Part model, mm, in its own coordinate system. Face numbers are marked on the shaded views. A direction names the side the tool comes from. Coordinates: 2 decimals unless noted, no trailing zeros. Loops run counter-clockwise (first coordinate to the right, second up) from the corner with the lowest first, then second, coordinate; pieces in that order, holes last. Notation, with made-up numbers: (-6.5, -26) - (51.5, -26) arc R12 cw to (51.5, -9) - close; hole circle Ø9 at (38, -3). An arc over 180 degrees is marked (long way). Use a Markdown table: item, result. Add a question column.
1. Wall check: probe 1 along Y at (x, z) = (0, 7.75); probe 2 along X at (y, z) = (-2.5, 7); probe 3 along X at (y, z) = (-8.5, 6.5). Give the ranges that are in metal, low to high. Write a range as [from, to].
2. Band-saw the part on D-D, the plane z = 7.5. Give the cut face in (x, y), plus the area to 3 significant figures.
3. Band-saw the part on B-B, the plane y = 0. Give the cut face in (x, z).
4. Pull direction X, two halves, no side cores. Call the marked faces 1, 2 and 3: pulls with the +X half, pulls with the -X half, needs draft (parallel to the pull), parting line crosses it, or undercut.
5. Band-saw the part on C-C, the plane z = 2.75. Give the cut face in (x, y).
6. Drop flat-ended pins along their axis: pin 1 (5 mm diameter, centred on x = 21, z = 3.5, fed in from +Y); pin 2 (1 mm diameter, centred on y = -18, z = 3.5, fed in from +X); pin 3 (23.5 mm diameter, centred on x = 0, y = 0, fed in from +Z). Give the stop position or say it passes through.
7. 3-axis set-ups, long thin cutter, end or side, ignore diameter. For the marked faces 4 and 5: which of +Z, -Z, +X, -X, +Y, -Y reach the whole face in a straight line?
8. Band-saw the part on A-A, the plane x = 0. Give the cut face in (y, z), plus the area to 3 significant figures.
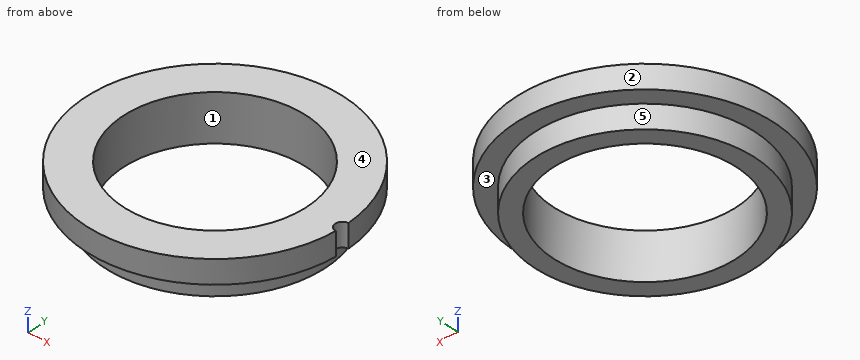
from build123d import *

# Parameters (mm, degrees)
SKETCH_R          = 27.5
SKETCH_R_2        = 19.5
PAD_DEPTH         = 10
SKETCH001_R       = 1.5
POCKET_DEPTH      = 10
SKETCH002_R       = 1.5
POCKET001_DEPTH   = 1.5
COPYSKETCH003_R   = 27.5
COPYSKETCH003_R_2 = 23.5
POCKET002_DEPTH   = 5


with BuildPart() as part:
    # Sketch → Pad (new body)
    with BuildSketch(Plane.XY):
        Circle(SKETCH_R)
        Circle(SKETCH_R_2, mode=Mode.SUBTRACT)
    extrude(amount=PAD_DEPTH)

    # Sketch001 → Pocket (cut)
    with BuildSketch(Plane(origin=(27.5, 0, 0), x_dir=(1, 0, 0), z_dir=(0, 0, 1))):
        Circle(SKETCH001_R)
    extrude(amount=POCKET_DEPTH, mode=Mode.SUBTRACT)

    # Sketch002 → Pocket001 (cut)
    with BuildSketch(Plane.YZ.offset(27.5)):
        Circle(SKETCH002_R)
    extrude(amount=-POCKET001_DEPTH, mode=Mode.SUBTRACT)

    # CopySketch003 → Pocket002 (cut)
    with BuildSketch(Plane.XY):
        Circle(COPYSKETCH003_R)
        Circle(COPYSKETCH003_R_2, mode=Mode.SUBTRACT)
    extrude(amount=POCKET002_DEPTH, mode=Mode.SUBTRACT)


solid = part.part
Geometry check:
| question | item | result |
|---|---|---|
| 1 | probe 1 | y = [-27.5, -19.5], [19.5, 27.5] |
| 1 | probe 2 | x = [-27.39, -19.34], [19.34, 27.39] |
| 1 | probe 3 | x = [-26.15, -17.55], [17.55, 26.15] |
| 2 | outline | (27.46, -1.5) arc R1.5 cw to (27.46, 1.5) arc R27.5 ccw (long way) to start; hole circle Ø39 at (0, 0) |
| 2 | area | 1,180 mm^2 |
| 3 | outline | (-27.5, 5) - (-23.5, 5) - (-23.5, 0) - (-19.5, 0) - (-19.5, 10) - (-27.5, 10) - close; (19.5, 0) - (23.5, 0) - (23.5, 5) - (26, 5) - (26, 10) - (19.5, 10) - close |
| 4 | face 1 | undercut |
| 4 | face 2 | parting line crosses it |
| 4 | face 3 | needs draft |
| 5 | outline | circle Ø47 at (0, 0); hole circle Ø39 at (0, 0) |
| 6 | pin 1 | stops at y = 19.88 |
| 6 | pin 2 | stops at x = 15.68 |
| 6 | pin 3 | passes through |
| 7 | face 4 | +Z, +X, -X, +Y, -Y |
| 7 | face 5 | -Z |
| 8 | outline | (-27.5, 5) - (-23.5, 5) - (-23.5, 0) - (-19.5, 0) - (-19.5, 10) - (-27.5, 10) - close; (19.5, 0) - (23.5, 0) - (23.5, 5) - (27.5, 5) - (27.5, 10) - (19.5, 10) - close |
| 8 | area | 120 mm^2 |
